Geometry: final body of the model. Coordinates: model frame, mm. Face numbers are marked on the shaded views. A direction names the side the tool comes from. Coordinates: 2 decimals unless noted, no trailing zeros. Loops run counter-clockwise (first coordinate to the right, second up) from the corner with the lowest first, then second, coordinate; pieces in that order, holes last. Notation, with made-up numbers: (10, 7.25) - (18, 7.25) arc R26 ccw to (18, 40.25) - close; hole circle Ø5 at (-31, -12.75). An arc over 180 degrees is marked (long way). Return JSON: item names as keys, results as strings.
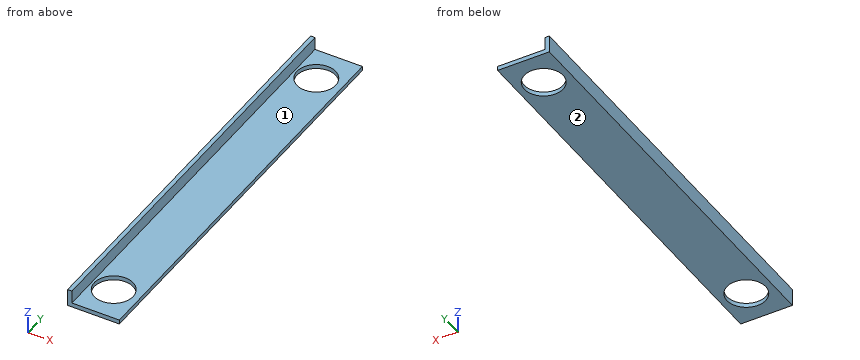
Autodesk Inventor part; units mm, degrees
ref_plane "YZ Plane" through (0, 0, 0) normal (1, 0, 0) x (0, 1, 0)
ref_plane "XZ Plane" through (0, 0, 0) normal (0, 1, 0) x (-1, 0, 0)
ref_plane "XY Plane" through (0, 0, 0) normal (0, 0, 1) x (1, 0, 0)
sketch "Sketch1" plane through (0, 0, 0) normal (0, 1, 0) x (-1, 0, 0)
  line L0 (14.0408, 9.525) -> (10.8658, 9.525)
  line L1 (-24.0592, 0) -> (-24.0592, -3.175)
  line L2 (-24.0592, -3.175) -> (14.0408, -3.175)
  line L3 (14.0408, -3.175) -> (14.0408, 9.525)
  line L4 (10.8658, 9.525) -> (10.8658, 0)
  line L5 (10.8658, 0) -> (-24.0592, 0)
  point P0 (0, 0)
  dimension "d0" = 38.1
  dimension "d1" = 12.7
  dimension "d2" = 3.175
  dimension "d3" = 3.175
extrude "Extrusion1" add sketch "Sketch1" along normal blind 304.8
sketch "Sketch2" plane through (-10.8658, 0, 0) normal (0, 0, 1) x (1, 0, 0)
  circle A0 centre (15.875, 25.4) radius 14.2875
  line L0 (34.925, 0) -> (34.925, 304.8)
  line L1 (0, 0) -> (34.925, 0)
  circle A1 centre (15.875, 279.4) radius 14.2875
  line L2 (0, 304.8) -> (34.925, 304.8)
  point P0 (10.8658, 0)
  dimension "d6" = 19.05
  dimension "d7" = 25.4
  dimension "d8" = 19.05
  dimension "d9" = 25.4
  dimension "d12" = 28.575
  dimension "d13" = 28.575
extrude "Extrusion2" cut sketch "Sketch2" against normal through all
equation "\"d10\" = d7"
properties part number "arm"
Item 1: Section query B-B, the plane x = 14. Return loops of the section in (y, z) (3 decimals).
Worked out:
{"outline": "(0, -3.175) - (14.296, -3.175) - (14.296, 0) - (0, 0) - close; (36.504, -3.175) - (268.296, -3.175) - (268.296, 0) - (36.504, 0) - close; (290.504, -3.175) - (304.8, -3.175) - (304.8, 0) - (290.504, 0) - close"}
Item 2: Section query D-D, the plane y = 154. Return loops of the section in (x, z) (3 decimals).
Worked out:
{"outline": "(-14.041, -3.175) - (24.059, -3.175) - (24.059, 0) - (-10.866, 0) - (-10.866, 9.525) - (-14.041, 9.525) - close"}
Item 3: Section query A-A, the plane y = 25.4. Return loops of the section in (x, z) (3 decimals).
Worked out:
{"outline": "(-14.041, -3.175) - (-9.278, -3.175) - (-9.278, 0) - (-10.866, 0) - (-10.866, 9.525) - (-14.041, 9.525) - close; (19.297, -3.175) - (24.059, -3.175) - (24.059, 0) - (19.297, 0) - close"}
Item 4: Ray query, probe 1 along Y at (x, z) = (4, -1.25); probe 2 along Y at (x, z) = (3.5, -0.5); probe 3 along Z at (x, y) = (9.5, 224.5) (3 decimals). Return the intervals inside material, ascending. Write a range as from..to.
Worked out:
{"probe 1": "0..11.15, 39.65..265.15, 293.65..304.8", "probe 2": "0..11.19, 39.61..265.19, 293.61..304.8", "probe 3": "-3.175..0"}
Item 5: Section query C-C, the plane x = -1.5. Return loops of the section in (y, z) (3 decimals), and give its area (3 significant figures).
Worked out:
{"outline": "(0, -3.175) - (12.681, -3.175) - (12.681, 0) - (0, 0) - close; (38.119, -3.175) - (266.681, -3.175) - (266.681, 0) - (38.119, 0) - close; (292.119, -3.175) - (304.8, -3.175) - (304.8, 0) - (292.119, 0) - close", "area": "806 mm^2"}
Item 6: First-contact query: pin 1 Ø2 at (x, y) = (-4.5, 215.5) entering from +Z; pin 2 Ø6 at (y, z) = (102.5, 6.5) entering from +X. Flat tips, straight axial feed; report the tip coordinate or a pass-through.
Worked out:
{"pin 1": "z = 0", "pin 2": "x = -10.87"}
Item 7: Reachability of the marked faces 1 and 2 from +Z, -Z, +X, -X, +Y, -Y: full face, straight path, thin tool, end or side. Return the list, or none.
Worked out:
{"face 1": "+Z, +X, +Y, -Y", "face 2": "-Z, +X, -X, +Y, -Y"}
